Drawing for the job (mm, zero at the part's lowest x, y, z). Give positions to 0.01 mm unless a question says otherwise; leave off trailing zeros. Order: outer loops, then holes, each group sorted by start corner. A loop starts at its lowest first (then second) coordinate and runs counter-clockwise, first axis right, second up. Notation, with made-up numbers: (-8.5, 2) -> (0.5, 2) arc R25 ccw to (0.5, 29) -> close; hole circle Ø5 at (46, 8). An arc over 180 degrees is marked (long way). One line per item, written item: value. Start each with the question number.
(1) Saw through at A-A on z = 3.75. Give the cut face in (x, y), plus the area to 3 significant figures.
(2) Probe line 1 (X direction, y = 3.2, z = 28.25). List the from-to ranges inside material, lowest first.
(3) Pin check, flat tips, straight feed: pin 1 (2 mm diameter, centred on x = 124, y = 1, fed in from -Z); pin 2 (2 mm diameter, centred on y = 2, z = 26.5, fed in from +X); pin 3 (2 mm diameter, centred on x = 316.5, y = 1.5, fed in from +Z); pin 4 (1.2 mm diameter, centred on x = 317, y = 2.5, fed in from -Z). Stop position of each tip, or through.
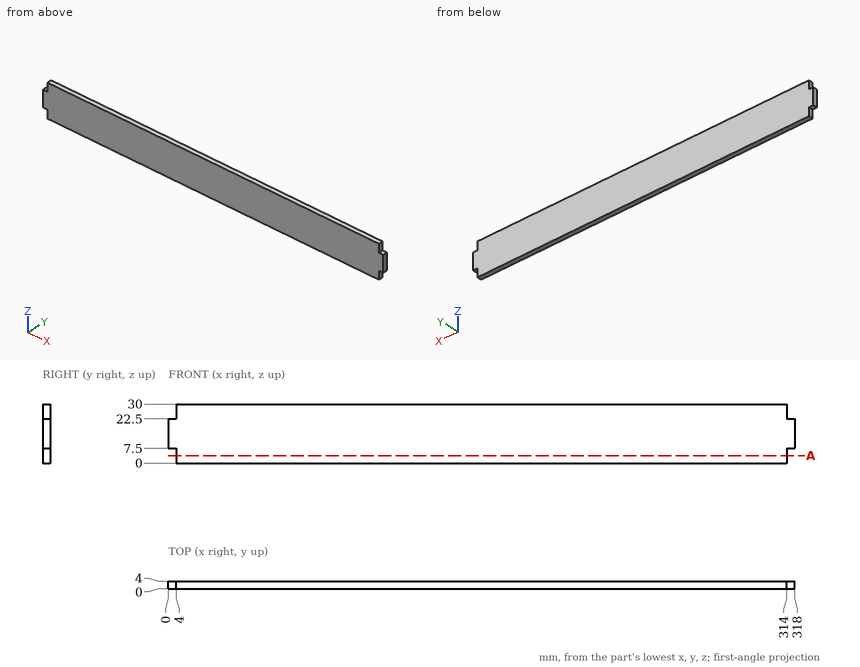
Results below:
1. outline: (4, 0) -> (314, 0) -> (314, 4) -> (4, 4) -> close
1. area: 1,240 mm²
2. line 1: x = 4 to 314
3. pin 1: stops at z = 0
3. pin 2: stops at x = 314
3. pin 3: stops at z = 22.5
3. pin 4: stops at z = 7.5
